from build123d import *

# Parameters (mm, degrees)
SKETCH1_R           = 1.65
SKETCH1_R_2         = 2.5
BOSS_EXTRUDE1_DEPTH = 2
BOSS_EXTRUDE2_DEPTH = 20
SKETCH4_W           = 1
SKETCH4_H           = 5
BOSS_EXTRUDE3_DEPTH = 22
SKETCH5_W           = 5
SKETCH5_H           = 1
BOSS_EXTRUDE4_DEPTH = 22
BOSS_EXTRUDE5_DEPTH = 2
CHAMFER1_SIZE       = 5
CHAMFER1_SIZE2      = 20


with BuildPart() as part:
    # Sketch1 → Boss-Extrude1 (new body)
    with BuildSketch(Plane(origin=(0, 0, 0), x_dir=(1, 0, 0), z_dir=(0, 1, 0))):
        Polygon((20, 18), (115, 18), (115, 42), (20, 42), (20, 60), (0, 60), (0, 0), (20, 0), align=None)
        with Locations(Location((10, 10, 0), (0, 0, 270))):
            Circle(SKETCH1_R, mode=Mode.SUBTRACT)
        with Locations(Location((10, 50, 0), (0, 0, 270))):
            Circle(SKETCH1_R, mode=Mode.SUBTRACT)
        with Locations(Location((103, 30, 0), (0, 0, 270))):
            Circle(SKETCH1_R_2, mode=Mode.SUBTRACT)
    extrude(amount=BOSS_EXTRUDE1_DEPTH)

    # Sketch2 → Boss-Extrude2 (add)
    with BuildSketch(Plane(origin=(0, 2, 0), x_dir=(1, 0, 0), z_dir=(0, 1, 0))):
        Polygon((115, 42), (93, 42), (93, 40), (100.5, 40), (100.5, 37), (105.5, 37), (105.5, 40), (113, 40), (113, 32.5), (110, 32.5), (110, 27.5), (113, 27.5), (113, 20), (105.5, 20), (105.5, 23), (100.5, 23), (100.5, 20), (93, 20), (93, 18), (115, 18), align=None)
    extrude(amount=BOSS_EXTRUDE2_DEPTH)

    # Sketch4 → Boss-Extrude3 (add)
    with BuildSketch(Plane(origin=(0, 0, 0), x_dir=(1, 0, 0), z_dir=(0, 1, 0))):
        with Locations((98.75, 15.5)):
            Rectangle(SKETCH4_W, SKETCH4_H)
        with Locations((93.5, 15.5)):
            Rectangle(SKETCH4_W, SKETCH4_H)
        with Locations((104, 15.5)):
            Rectangle(SKETCH4_W, SKETCH4_H)
        with Locations((109.25, 15.5)):
            Rectangle(SKETCH4_W, SKETCH4_H)
        with Locations((114.5, 15.5)):
            Rectangle(SKETCH4_W, SKETCH4_H)
        with Locations((114.5, 44.5)):
            Rectangle(SKETCH4_W, SKETCH4_H)
        with Locations((109.25, 44.5)):
            Rectangle(SKETCH4_W, SKETCH4_H)
        with Locations((104, 44.5)):
            Rectangle(SKETCH4_W, SKETCH4_H)
        with Locations((98.75, 44.5)):
            Rectangle(SKETCH4_W, SKETCH4_H)
        with Locations((93.5, 44.5)):
            Rectangle(SKETCH4_W, SKETCH4_H)
    extrude(amount=BOSS_EXTRUDE3_DEPTH)

    # Sketch5 → Boss-Extrude4 (add)
    with BuildSketch(Plane(origin=(0, 0, 0), x_dir=(1, 0, 0), z_dir=(0, 1, 0))):
        with Locations((117.5, 18.5)):
            Rectangle(SKETCH5_W, SKETCH5_H)
        with Locations((117.5, 24.25)):
            Rectangle(SKETCH5_W, SKETCH5_H)
        with Locations((117.5, 30)):
            Rectangle(SKETCH5_W, SKETCH5_H)
        with Locations((117.5, 35.75)):
            Rectangle(SKETCH5_W, SKETCH5_H)
        with Locations((117.5, 41.5)):
            Rectangle(SKETCH5_W, SKETCH5_H)
    extrude(amount=BOSS_EXTRUDE4_DEPTH)

    # Sketch6 → Boss-Extrude5 (add)
    with BuildSketch(Plane(origin=(0, 0, 0), x_dir=(1, 0, 0), z_dir=(0, 1, 0))):
        Polygon((90, 42), (115, 42), (115, 18), (90, 18), (93, 13), (115, 13), (120, 18), (120, 42), (115, 47), (93, 47), align=None)
    extrude(amount=BOSS_EXTRUDE5_DEPTH)

    # Chamfer1
    chamfer1_edges = [part.edges().sort_by_distance(p)[0] for p in [
        (93.5, 22, -47),
        (98.75, 22, -47),
        (104, 22, -47),
        (109.25, 22, -47),
        (120, 22, -41.5),
        (120, 22, -35.75),
        (120, 22, -30),
        (120, 22, -18.5),
        (114.5, 22, -13),
        (109.25, 22, -13),
        (104, 22, -13),
        (98.75, 22, -13),
        (114.5, 22, -47),
        (120, 22, -24.25),
        (93.5, 22, -13),
    ]]
    chamfer1_side = [part.faces().sort_by_distance(p)[0] for p in [
        (93.565834133, 22, -15.5),
    ]]
    chamfer(chamfer1_edges, length=CHAMFER1_SIZE, length2=CHAMFER1_SIZE2, reference=chamfer1_side[0])


solid = part.part
CAD build for the part. Positions are in the model's coordinates, mm. A direction names the side the tool comes from. Coordinates: 2 decimals unless noted, no trailing zeros. Write each loop counter-clockwise with the first axis right and the second up, starting at its lowest first coordinate (ties: lowest second). Pieces come first, ordered by that corner, then holes. Notation, with made-up numbers: M 83.25,75.5 L 102.25,75.5 A34 cw 102.25,109.5 Z; hole C 19.25,-4 d9. An arc over 180 degrees is marked long. Answer as a JSON object with one key per item and string values. Group by question number.
1) Saw through at A-A (z = -10). Write the cut outline in (x, y), plus the area to 3 significant figures.
2) Tool access for faces 5 (the face through (105.48, 0.99, -30.33)), 6 (the face through (116, 2, -43)), 7 (the face through (115, 12, -21)), 8 (the face through (104.5, 7, -17)), 9 (the face through (101, 2, -45)): list every direction of +Z, -Z, +X, -X, +Y, -Y with a clear straight run to the whole face (end or side of a thin tool).
3) Saw through at C-C (x = 96). Write the cut outline in (y, z).
4) Saw through at D-D (x = 57.5). Write the cut outline in (y, z), plus the area to 3 significant figures.
5) Saw through at B-B (x = 10). Write the cut outline in (y, z).
6) Wall check: line 1 (X direction, y = 1.05, z = -10); line 2 (Z direction, x = 96, y = 9.5); line 3 (X direction, y = 1.3, z = -30). Give the ranges that are in metal, low to high. Write a range as from..to.
7) Mould opens along Z. For faces 1 (the face through (98.25, 10, -44)), 2 (the face through (111, 12, -27.5)), 3 (the face through (107, 12, -18)), 4 (the face through (105.5, 12, -21)) say: +Z half, -Z half, draft (parallel to the pull), parting line (faces both ways), or undercut.
8) Pin check, flat tips, straight feed: pin 1 Ø1.4 at (x, z) = (118.5, -26.5) entering from +Y; pin 2 Ø2.5 at (y, z) = (10, -45.5) entering from -X; pin 3 Ø2 at (x, z) = (10, -10) entering from +Y; pin 4 Ø4.5 at (x, y) = (112, 10) entering from +Z. Stop position of each tip, or through.
Values follow:
{
 "1": {"outline": "M 0,0 L 8.35,0 L 8.35,2 L 0,2 Z; M 11.65,0 L 20,0 L 20,2 L 11.65,2 Z", "area": "33.4 mm2"},
 "2": {"face 5": "+Y, -Y", "face 6": "-Z, +X, +Y", "face 7": "+X, +Y", "face 8": "+Z, +Y", "face 9": "-Z, +Y"},
 "3": {"outline": "M 0,-47 L 2,-47 L 2,-42 L 22,-42 L 22,-40 L 2,-40 L 2,-20 L 22,-20 L 22,-18 L 2,-18 L 2,-13 L 0,-13 Z"},
 "4": {"outline": "M 0,-42 L 2,-42 L 2,-18 L 0,-18 Z", "area": "48.0 mm2"},
 "5": {"outline": "M 0,-60 L 2,-60 L 2,-51.65 L 0,-51.65 Z; M 0,-48.35 L 2,-48.35 L 2,-11.65 L 0,-11.65 Z; M 0,-8.35 L 2,-8.35 L 2,0 L 0,0 Z"},
 "6": {"line 1": "x = 0..8.35, 11.65..20", "line 2": "z = -42..-40, -20..-18", "line 3": "x = 0..100.5, 105.5..120"},
 "7": {"face 1": "draft", "face 2": "undercut", "face 3": "+Z half", "face 4": "undercut"},
 "8": {"pin 1": "stops at y = 2", "pin 2": "stops at x = 93", "pin 3": "passes through", "pin 4": "stops at z = -14.74"}
}
